```python
from build123d import *

# Parameters (mm, degrees)
SKETCH_2_R          = 0.5
EXTRUDE_1_DEPTH     = 10
SKETCH_3_R          = 0.5
EXTRUDE_2_DEPTH     = 10
SKETCH_4_R          = 0.5
EXTRUDE_3_DEPTH     = 10
CUT_EXTRUDE_1_DEPTH = 1
CUT_EXTRUDE_2_DEPTH = 1
CUT_EXTRUDE_3_DEPTH = 1


with BuildPart() as part:
    # 草图1 → 旋转1 (revolve)
    with BuildSketch(Plane.XY):
        with BuildLine():
            Line((0, 1), (0, -1))
            ThreePointArc((0, -1), (-1, 0), (0, 1))
        make_face()
    revolve(axis=Axis((0, 1, 0), (0, -1, 0)))

    # 草图2 → 凸台-拉伸1 (add)
    with BuildSketch(Plane(origin=(0, 0, 0), x_dir=(1, 0, 0), z_dir=(0, 1, 0))):
        Circle(SKETCH_2_R)
    extrude(amount=EXTRUDE_1_DEPTH)

    # 草图3 → 凸台-拉伸2 (add)
    with BuildSketch(Plane(origin=(0, 0, 0), x_dir=(0, 0, -1), z_dir=(1, 0, 0))):
        Circle(SKETCH_3_R)
    extrude(amount=EXTRUDE_2_DEPTH)

    # 草图4 → 凸台-拉伸3 (add)
    with BuildSketch(Plane.XY):
        Circle(SKETCH_4_R)
    extrude(amount=EXTRUDE_3_DEPTH)

    # 草图5 → 切除-拉伸1 (cut)
    with BuildSketch(Plane.XY.offset(10)):
        Polygon((0.164271664, -0.305303511), (0.080061137, -0.305303511), (-0.039237108, -0.059689476), (-0.158535354, -0.305303511), (-0.24274588, -0.305303511), (-0.0778336, 0.010485963), (-0.225202021, 0.294696489), (-0.140991494, 0.294696489), (-0.039237108, 0.07715263), (0.062517278, 0.294696489), (0.146727804, 0.294696489), (-0.000640617, 0.010485963), align=None)
    extrude(amount=-CUT_EXTRUDE_1_DEPTH, mode=Mode.SUBTRACT)

    # 草图6 → 切除-拉伸2 (cut)
    with BuildSketch(Plane(origin=(10, 0, 0), x_dir=(0, 0, -1), z_dir=(1, 0, 0))):
        Polygon((0.196855421, 0.324059335), (0.03194314, -0.005765227), (0.03194314, -0.275940665), (-0.048758614, -0.275940665), (-0.048758614, -0.005765227), (-0.213670895, 0.324059335), (-0.13296914, 0.324059335), (-0.010162123, 0.067918984), (-0.006653351, 0.067918984), (0.116153667, 0.324059335), align=None)
    extrude(amount=-CUT_EXTRUDE_2_DEPTH, mode=Mode.SUBTRACT)

    # 草图7 → 切除-拉伸3 (cut)
    with BuildSketch(Plane(origin=(0, 10, 0), x_dir=(1, 0, 0), z_dir=(0, 1, 0))):
        Polygon((0.164917999, -0.276228525), (-0.210520598, -0.276228525), (-0.210520598, -0.209561858), (0.073689928, 0.257104808), (-0.189467966, 0.257104808), (-0.189467966, 0.323771475), (0.154391683, 0.323771475), (0.154391683, 0.257104808), (-0.129818843, -0.209561858), (0.164917999, -0.209561858), align=None)
    extrude(amount=-CUT_EXTRUDE_3_DEPTH, mode=Mode.SUBTRACT)


solid = part.part
```
Can you work these out from the model? Positions are in its coordinate system, mm. A direction names the side the tool comes from. Round coordinates to 2 decimals unless told otherwise and drop trailing zeros. Loops run counter-clockwise (first coordinate to the right, second up) from the corner with the lowest first, then second, coordinate; pieces in that order, holes last. Notation, with made-up numbers: (-39.5, 74) -> (-28.5, 74) arc R22 cw to (-28.5, 84) -> close; hole circle Ø5 at (83.5, 69.5). An arc over 180 degrees is marked (long way). Answer in a Markdown table with one row per item.
Item 1: Suppose I cut it at A-A, the plane y = 2.75. List the corners of the cut face in (x, z) for me.
Answer block:
| item | result |
|---|---|
| outline | circle Ø1 at (0, 0) |
Item 2: If I drill on probe 1 along Y at (x, z) = (0, 1); probe 2 along Z at (x, y) = (3, 0.25), over which ranges is the centre line in solid material (lowest first)?
Answer block:
| item | result |
|---|---|
| probe 1 | -0.5 to 0.5 |
| probe 2 | -0.43 to 0.43 |
Item 3: On a 3-axis mill with a long thin cutter (end or side, diameter ignored), from which of +Z, -Z, +X, -X, +Y, -Y can I reach the whole of each face in a straight line? I mean faces 1 (the flat face through (0.2, 0, 10)), 2 (the cylindrical face through (5.369, -0.488, 0.108)), 3 (the cylindrical face through (-0.108, -0.488, 5.369)), 4 (the cylindrical face through (-0.108, 5.369, 0.488)). Say none if no direction works.
Answer block:
| item | result |
|---|---|
| face 1 | +Z, +X, -X, +Y, -Y |
| face 2 | +X |
| face 3 | +Z |
| face 4 | +Y |
Item 4: Will these pins go through, and if not, where does the flat tip stop? P1, Ø4, axis at x = 1, z = 2.5, coming from the +Y side; P2, Ø3, axis at y = 1, z = 8.5, coming from the -X side; P3, Ø1, axis at x = 0.5, y = 2.5, coming from the -Z side.
Answer block:
| item | result |
|---|---|
| P1 | y = 0.72 |
| P2 | x = -0.5 |
| P3 | z = -0.5 |
